Autodesk Inventor part; units mm, degrees
ref_plane "YZ Plane" through (0, 0, 0) normal (1, 0, 0) x (0, 1, 0)
ref_plane "XZ Plane" through (0, 0, 0) normal (0, 1, 0) x (-1, 0, 0)
ref_plane "XY Plane" through (0, 0, 0) normal (0, 0, 1) x (1, 0, 0)
sketch "Sketch1" plane through (0, 0, 0) normal (0, 0, 1) x (1, 0, 0)
  circle A0 centre (0, 0) radius 2.175
  circle A1 centre (0, 0) radius 1.75
  circle A2 centre (0, 0) radius 2.875
  circle A3 centre (0, 0) radius 2.25
  dimension "d0" = 4.35
  dimension "d1" = 3.5
  dimension "d2" = 5.75
  dimension "d3" = 4.5
extrude "Extrusion1" add sketch "Sketch1" along normal blind 81.5 contours A0 | A1
extrude "Extrusion2" add sketch "Sketch1" against normal blind 2 contours A0 | A1 | A2 | A3
fillet "Fillet1" radius 1 1 edges at (-2.875, 0, -2)
sketch "Sketch2" plane through (0, 0, 81.5) normal (0, 0, 1) x (1, 0, 0)
  circle A0 centre (0, 0) radius 1.75
  dimension "d9" = 3.5
extrude "Extrusion3" cut sketch "Sketch2" against normal blind 20
properties part number "Schanier pin"
Could you check a few things on this model? Use its own coordinates, in mm. A direction names the side the tool comes from. Coordinates: 2 decimals unless noted, no trailing zeros. Order: outer loops, then holes, each group sorted by start corner. A loop starts at its lowest first (then second) coordinate and runs counter-clockwise, first axis right, second up. Notation, with made-up numbers: M -11,55 L 6,55 A22 cw 6,78 Z; hole C 25,-38.5 d5. An arc over 180 degrees is marked long. Use one line per item in the form item = value. Start each with the question number.
1. On a 3-axis mill with a long thin cutter (end or side, diameter ignored), from which of +Z, -Z, +X, -X, +Y, -Y can I reach the whole of each face in a straight line? I mean faces 1 (the flat face through (0, 2, 81.5)), 2 (the flat face through (0, 0, 61.5)). Say none if no direction works.
2. For pin 1 (3 mm diameter, centred on x = 0, y = 0, fed in from +Z); pin 2 (3 mm diameter, centred on x = -1.5, z = 16, fed in from +Y) (3 decimals); pin 3 (2 mm diameter, centred on y = -2, z = 66.5, fed in from -X), each with a flat end and sliding along its axis, tell me the tip position at first contact or that it passes through.
3. Suppose I cut it at A-A on x = 0. Write out the boundary of the cut face in (y, z) (3 decimals), then the cut area to 3 significant figures.
4. Suppose I cut it at C-C on z = 64.5. Write out the boundary of the cut face in (x, y) (3 decimals).
5. Suppose I cut it at D-D on z = 44.5. Write out the boundary of the cut face in (x, y) (3 decimals).
6. We'd pull the mould along X, two halves only. Please class faces 3 (the cylindrical face through (1.617, -0.67, 71.64)), 4 (the flat face through (0, 0, -2)), 5 (the cylindrical face through (-0.37, 2.85, -0.49)): +X half, -X half, draft (parallel to the pull), parting line (faces both ways), or undercut.
7. Please list where these lines run through material, in increasing order: line 1 (Y direction, x = 0, z = 67.5) (3 decimals); line 2 (Z direction, x = 1.55, y = -0.5); line 3 (Z direction, x = -0.9, y = -2.2).
Geometry says:
q1.face_1 = +Z, +X, -X, +Y, -Y
q1.face_2 = +Z
q2.pin_1 = 61.5
q2.pin_2 = 2.175
q2.pin_3 = -1.93
q3.outline = M -2.875,-1 A1 ccw -1.875,-2 L 1.875,-2 A1 ccw 2.875,-1 L 2.875,0 L 2.175,0 L 2.175,81.5 L 1.75,81.5 L 1.75,61.5 L -1.75,61.5 L -1.75,81.5 L -2.175,81.5 L -2.175,0 L -2.875,0 Z
q3.area = 296 mm^2
q4.outline = C 0,0 d4.35; hole C 0,0 d3.5
q5.outline = C 0,0 d4.35
q6.face_3 = undercut
q6.face_4 = draft
q6.face_5 = parting line
q7.line_1 = -2.175 to -1.75, 1.75 to 2.175
q7.line_2 = -2 to 61.5
q7.line_3 = -1.86 to 0
